from build123d import *

# Parameters (mm, degrees)
ESBO_O1_R                                   = 3
RESSALTO_EXTRUS_O1_DEPTH                    = 85
BROCA_DE_ROSQUEAR_PARA_TARRAXA_DE_M32_D     = 2.5
BROCA_DE_ROSQUEAR_PARA_TARRAXA_DE_M32_DEPTH = 8
BROCA_DE_ROSQUEAR_PARA_TARRAXA_DE_M32_TIP   = 0.751075774


with BuildPart() as part:
    # Esboço1 → Ressalto-extrusão1 (new body)
    with BuildSketch(Plane.XY):
        Circle(ESBO_O1_R)
    extrude(amount=RESSALTO_EXTRUS_O1_DEPTH)

    # Esboço2 → Broca de rosquear para tarraxa de M31 (revolve, cut)
    with BuildSketch(Plane(origin=(0, 0, 85), x_dir=(0, -1, 0), z_dir=(1, 0, 0))):
        Polygon((0, 0), (0, 8.751075774), (1.25, 8), (1.25, 0), align=None)
    revolve(axis=Axis((0, 0, 91.35), (0, 0, -1)), mode=Mode.SUBTRACT)

    # Broca de rosquear para tarraxa de M32
    with Locations(Plane(origin=(0, 0, 0), x_dir=(-1, 0, 0), z_dir=(0, 0, -1))):
        with Locations((0, 0)):
            Hole(BROCA_DE_ROSQUEAR_PARA_TARRAXA_DE_M32_D / 2, depth=BROCA_DE_ROSQUEAR_PARA_TARRAXA_DE_M32_DEPTH)
            with Locations((0, 0, -(BROCA_DE_ROSQUEAR_PARA_TARRAXA_DE_M32_DEPTH + BROCA_DE_ROSQUEAR_PARA_TARRAXA_DE_M32_TIP / 2))):  # 118° drill point
                Cone(0, BROCA_DE_ROSQUEAR_PARA_TARRAXA_DE_M32_D / 2, BROCA_DE_ROSQUEAR_PARA_TARRAXA_DE_M32_TIP, mode=Mode.SUBTRACT)


solid = part.part
Read the model definition and answer for the solid it produces. Units are mm, in the model's axes. A direction names the side the tool comes from. Coordinates: 2 decimals unless noted, no trailing zeros. Loops run counter-clockwise (first coordinate to the right, second up) from the corner with the lowest first, then second, coordinate; pieces in that order, holes last.
Q1. Which of the six approach directions +Z, -Z, +X, -X, +Y, -Y give full straight-line access (tool end or side, diameter ignored) to faces 5 (the face through (1, -1, 85)), 6 (the face through (-0.27, -1.22, 4.06))?
Q2. Consider probe 1 along Y at (x, z) = (0, 3.75); probe 2 along Y at (x, z) = (0.95, 78); probe 3 along Y at (x, z) = (-1.75, 32.5). Determine where each line is inside the solid, lowest interval first.
Q3. The part is cut by section C-C on x = 1.95. Write down the section's boundary in (y, z).
Q4. The mould has two halves that part along Y. Classify faces 1 (the face through (1.22, 0.27, 81.06)), 2 (the face through (1, -1, 0)), 3 (the face through (0.05, -0.21, 8.62)), 4 (the face through (-3, 0, 42)): +Y half, -Y half, draft (parallel to the pull), parting line (faces both ways), or undercut.
Q5. Each of these flat-tipped pins is pushed along its axis until it touches: pin 1 Ø1.5 at (x, z) = (-1.5, 73.5) entering from +Y; pin 2 Ø2 at (x, y) = (0, 0) entering from -Z. Where does it stop, or does it pass through?
Q6. The part is cut by section A-A on z = 72. Write down the section's boundary in (x, y), and give its area (3 significant figures).
Q7. The part is cut by section B-B on y = 2.3. Write down the section's boundary in (x, z), and give its area (3 significant figures).
Results below:
1. face 5: +Z, +X, -X, +Y, -Y
1. face 6: -Z
2. probe 1: y = -3 to -1.25, 1.25 to 3
2. probe 2: y = -2.85 to -0.81, 0.81 to 2.85
2. probe 3: y = -2.44 to 2.44
3. outline: (-2.28, 0) - (2.28, 0) - (2.28, 85) - (-2.28, 85) - close
4. face 1: undercut
4. face 2: draft
4. face 3: undercut
4. face 4: parting line
5. pin 1: stops at y = 2.9
5. pin 2: stops at z = 8.15
6. outline: circle Ø6 at (0, 0)
6. area: 28.3 mm2
7. outline: (-1.93, 0) - (1.93, 0) - (1.93, 85) - (-1.93, 85) - close
7. area: 327 mm2
